The listing builds one solid part. Answer for the finished solid, in the listing's coordinates (mm). Face numbers are marked on the shaded views. A direction names the side the tool comes from. Give positions to 0.01 mm unless a question says otherwise; leave off trailing zeros. Loops run counter-clockwise (first coordinate to the right, second up) from the corner with the lowest first, then second, coordinate; pieces in that order, holes last. Notation, with made-up numbers: (72.5, 33.5) - (91.5, 33.5) arc R28 ccw to (91.5, 52.5) - close; hole circle Ø4 at (-6, 53.5). An arc over 180 degrees is marked (long way). Answer in a Markdown table with one row per item. Add a question column.
```python
from build123d import *

# Parameters (mm, degrees)
F0_R          = 38.1
F1_DEPTH      = 15.875
F1_DEPTH_BACK = 15.875
F3_DEPTH      = 25.4
F4_DEPTH      = 25.4
F6_DEPTH      = 25.4
F7_R          = 12.7
F8_DEPTH      = 25.4
F10_DEPTH     = 152.4


with BuildPart() as f1:
    # F0 (on Right) → F1 (new body, two sides)
    with BuildSketch(Plane.YZ) as f1_sk:
        with BuildLine():
            Line((114.3, 76.2), (0, 76.2))
            ThreePointArc((0, 76.2), (-76.2, 0), (0, -76.2))
            Line((0, -76.2), (114.3, -76.2))
            Line((114.3, -76.2), (114.3, -50.8))
            Line((114.3, -50.8), (88.9, -50.8))
            Line((88.9, -50.8), (88.9, 50.8))
            Line((88.9, 50.8), (114.3, 50.8))
            Line((114.3, 50.8), (114.3, 76.2))
        make_face()
        Circle(F0_R, mode=Mode.SUBTRACT)
    extrude(amount=F1_DEPTH)
    extrude(f1_sk.sketch, amount=-F1_DEPTH_BACK)

    # F2 (on face) → F3 (join, through all)
    with BuildSketch(Plane.XY.offset(76.2)):
        with BuildLine():
            Line((15.875, 114.3), (15.875, 107.172131))
            ThreePointArc((15.875, 107.172131), (0, 152.4), (-15.875, 107.172131))
            Line((-15.875, 107.172131), (-15.875, 114.3))
            Line((-15.875, 114.3), (0, 114.3))
            Line((0, 114.3), (15.875, 114.3))
        make_face()
        with BuildLine():
            ThreePointArc((12.7, 127), (8.980256, 118.019744), (0, 114.3))
            ThreePointArc((0, 114.3), (-8.980256, 135.980256), (12.7, 127))
        make_face(mode=Mode.SUBTRACT)
        with BuildLine():
            ThreePointArc((12.7, 127), (-8.980256, 135.980256), (0, 114.3))
            ThreePointArc((0, 114.3), (8.980256, 118.019744), (12.7, 127))
        make_face()
    extrude(amount=-F3_DEPTH)

    # F2 (on face) → F4 (cut, through all)
    with BuildSketch(Plane.XY.offset(76.2)):
        with BuildLine():
            ThreePointArc((12.7, 127), (-8.980256, 135.980256), (0, 114.3))
            ThreePointArc((0, 114.3), (8.980256, 118.019744), (12.7, 127))
        make_face()
    extrude(amount=-F4_DEPTH, mode=Mode.SUBTRACT)

    # F5 (on face) → F6 (join, through all)
    with BuildSketch(Plane.XY.offset(-50.8)):
        with BuildLine():
            Line((15.875, 114.3), (15.875, 107.172131))
            ThreePointArc((15.875, 107.172131), (0, 152.4), (-15.875, 107.172131))
            Line((-15.875, 107.172131), (-15.875, 114.3))
            Line((-15.875, 114.3), (15.875, 114.3))
        make_face()
    extrude(amount=-F6_DEPTH)

    # F7 (on face) → F8 (cut, through all)
    with BuildSketch(Plane.XY.offset(-50.8)):
        with Locations((0, 127)):
            Circle(F7_R)
    extrude(amount=-F8_DEPTH, mode=Mode.SUBTRACT)

    # F9 (on face) → F10 (cut, through all)
    with BuildSketch(Plane.XY.offset(76.2)):
        with BuildLine():
            Line((6.35, 12.7), (6.35, 63.5))
            ThreePointArc((6.35, 63.5), (0, 69.85), (-6.35, 63.5))
            Line((-6.35, 63.5), (-6.35, 12.7))
            ThreePointArc((-6.35, 12.7), (0, 6.35), (6.35, 12.7))
        make_face()
    extrude(amount=-F10_DEPTH, mode=Mode.SUBTRACT)


solid = f1.part
```
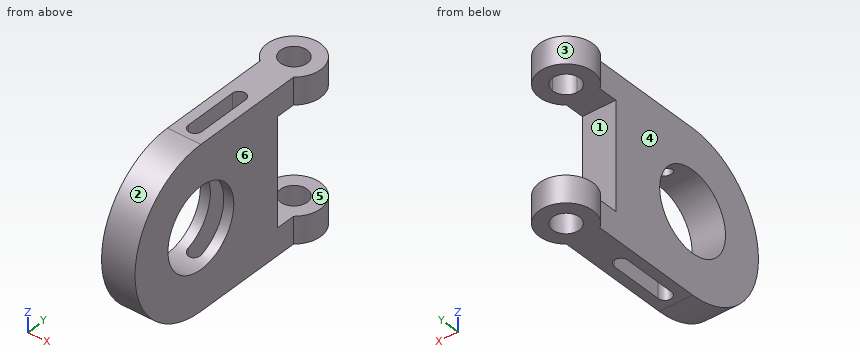
(1) A tool of negligible diameter and unlimited length cuts with its end or side. For the marked faces 4, 5 and 6, from which of +Z, -Z, +X, -X, +Y, -Y can it reach the whole face along a straight path? Write none if from no direction.
(2) A cutting plane is placed at B-B on x = 9. Determine the outline of the cut face in (y, z), plus the area to 3 significant figures.
(3) A cutting plane is placed at D-D on z = 45. Determine the outline of the cut face in (x, y) (3 decimals), plus the area to 3 significant figures.
(4) A cutting plane is placed at A-A on z = 0. Determine the outline of the cut face in (x, y) (3 decimals), plus the area to 3 significant figures.
(5) The mould has two halves that part along Z. Classify the marked faces 1, 2 and 3: pulls with the +Z half, pulls with the -Z half, needs draft (parallel to the pull), parting line crosses it, or undercut.
(6) Find the intervals of material crossed by line 1 along X through (y, z) = (24, -63.5) (3 decimals); line 2 along X through (y, z) = (127, 70.75); line 3 along Z through (x, y) = (-14, 104), in increasing order. Write a range as [from, to].
(7) Given pin 1 Ø12 at (x, z) = (-7, -6) entering from +Y; pin 2 Ø4 at (y, z) = (47.5, -4) entering from -X (3 decimals); pin 3 Ø6 at (x, z) = (1.5, -16.5) entering from -Y, each flat-ended and moving along its own axis, determine where each tip first touches the part or whether it passes through.
(8) A cutting plane is placed at C-C on y = -5.5. Determine the outline of the cut face in (x, z) (3 decimals), plus the area to 3 significant figures.
Evaluation:
| question | item | result |
|---|---|---|
| 1 | face 4 | +Z, -Z, -X, -Y |
| 1 | face 5 | +X, -X, +Y |
| 1 | face 6 | +Z, -Z, +X, -Y |
| 2 | outline | (0, -76.2) - (118.04, -76.2) - (118.04, -50.8) - (88.9, -50.8) - (88.9, 50.8) - (118.04, 50.8) - (118.04, 76.2) - (0, 76.2) arc R76.2 ccw to start; (135.96, -76.2) - (150.75, -76.2) - (150.75, -50.8) - (135.96, -50.8) - close; (135.96, 50.8) - (150.75, 50.8) - (150.75, 76.2) - (135.96, 76.2) - close; hole circle Ø76.2 at (0, 0) |
| 2 | area | 20,300 mm² |
| 3 | outline | (-15.875, -61.493) - (15.875, -61.493) - (15.875, 88.9) - (-15.875, 88.9) - close; hole (-6.35, 12.7) arc R6.35 ccw to (6.35, 12.7) - (6.35, 63.5) arc R6.35 ccw to (-6.35, 63.5) - close |
| 3 | area | 4,000 mm² |
| 4 | outline | (-15.875, -76.2) - (15.875, -76.2) - (15.875, -38.1) - (-15.875, -38.1) - close; (-15.875, 38.1) - (-6.35, 38.1) - (-6.35, 63.5) arc R6.35 cw to (6.35, 63.5) - (6.35, 38.1) - (15.875, 38.1) - (15.875, 88.9) - (-15.875, 88.9) - close |
| 4 | area | 2,440 mm² |
| 5 | face 1 | undercut |
| 5 | face 2 | parting line crosses it |
| 5 | face 3 | needs draft |
| 6 | line 1 | x = [-15.875, -6.35], [6.35, 15.875] |
| 6 | line 2 | x = [-25.4, -12.7], [12.7, 25.4] |
| 6 | line 3 | z = [-76.2, -50.8], [50.8, 76.2] |
| 7 | pin 1 | stops at y = 88.9 |
| 7 | pin 2 | stops at x = -15.875 |
| 7 | pin 3 | stops at y = -74.99 |
| 8 | outline | (-15.875, -76.001) - (15.875, -76.001) - (15.875, -37.701) - (-15.875, -37.701) - close; (-15.875, 37.701) - (15.875, 37.701) - (15.875, 76.001) - (-15.875, 76.001) - close |
| 8 | area | 2,430 mm² |
